```python
from build123d import *

# Parameters (mm, degrees)
BOSS_EXTRUDE1_DEPTH = 20
SKETCH2_R           = 26
CUT_EXTRUDE1_DEPTH  = 5
SKETCH3_R           = 30
CUT_EXTRUDE2_DEPTH  = 11
CUT_EXTRUDE3_DEPTH  = 187.815416923
FILLET1_R           = 6
CHAMFER1_SIZE       = 2
SKETCH6_W           = 10
SKETCH6_H           = 80
CUT_EXTRUDE4_DEPTH  = 5
CHAMFER2_SIZE       = 2
SKETCH7_R           = 10
SKETCH7_R_2         = 20
CUT_EXTRUDE5_DEPTH  = 5
CHAMFER3_SIZE       = 2


with BuildPart() as part:
    # Sketch1 → Boss-Extrude1 (new, symmetric)
    with BuildSketch(Plane.XY):
        with BuildLine():
            Line((-29.941348918, -1.875), (-19.960899278, -161.25))
            ThreePointArc((-19.960899278, -161.25), (0, -180), (19.960899278, -161.25))
            Line((19.960899278, -161.25), (29.941348918, -1.875))
            ThreePointArc((29.941348918, -1.875), (0, 30), (-29.941348918, -1.875))
        make_face()
    extrude(amount=BOSS_EXTRUDE1_DEPTH, both=True)

    # Sketch2 → Cut-Extrude1 (cut)
    with BuildSketch(Plane(origin=(0, 0, -20), x_dir=(-1, 0, 0), z_dir=(0, 0, -1))):
        Circle(SKETCH2_R)
    extrude(amount=-CUT_EXTRUDE1_DEPTH, mode=Mode.SUBTRACT)

    # Sketch3 → Cut-Extrude2 (cut, symmetric)
    with BuildSketch(Plane.XY):
        with Locations((0, -160)):
            Circle(SKETCH3_R)
    extrude(amount=CUT_EXTRUDE2_DEPTH, both=True, mode=Mode.SUBTRACT)

    # Sketch4 → Cut-Extrude3 (cut, through all)
    with BuildSketch(Plane(origin=(0, 0, -20), x_dir=(-1, 0, 0), z_dir=(0, 0, -1))):
        with BuildLine():
            ThreePointArc((-20.17601335, -29.814903745), (0, -36), (20.17601335, -29.814903745))
            Line((20.17601335, -29.814903745), (14.361387571, -122.667031366))
            ThreePointArc((14.361387571, -122.667031366), (0, -120), (-14.361387571, -122.667031366))
            Line((-14.361387571, -122.667031366), (-20.17601335, -29.814903745))
        make_face()
    extrude(amount=-CUT_EXTRUDE3_DEPTH, mode=Mode.SUBTRACT)

    # Fillet1
    fillet1_edges = [part.edges().sort_by_distance(p)[0] for p in [
        (20.17601335, -29.814903745, 0),
        (-20.17601335, -29.814903745, 0),
        (-14.361387571, -122.667031366, 0),
        (14.361387571, -122.667031366, 0),
    ]]
    fillet(fillet1_edges, radius=FILLET1_R)

    # Chamfer1
    chamfer1_edges = [part.edges().sort_by_distance(p)[0] for p in [
        (0, -180, 20),
        (24.951124098, -81.5625, 20),
        (0, 30, 20),
        (24.951124098, -81.5625, -20),
        (0, -120, -20),
        (0, -120, 20),
        (17.178453178, -77.682101085, -20),
        (0, -180, -20),
        (17.178453178, -77.682101085, 20),
        (-17.178453178, -77.682101085, -20),
        (-17.178453178, -77.682101085, 20),
        (-24.951124098, -81.5625, -20),
        (0, -36, -20),
        (0, -36, 20),
        (12.505327982, -119.60645162, -20),
        (12.505327982, -119.60645162, 20),
        (-12.505327982, -119.60645162, -20),
        (-12.505327982, -119.60645162, 20),
        (17.184830058, -34.989739942, -20),
        (0, 30, -20),
        (17.184830058, -34.989739942, 20),
        (-17.184830058, -34.989739942, -20),
        (-17.184830058, -34.989739942, 20),
        (-24.951124098, -81.5625, 20),
    ]]
    chamfer(chamfer1_edges, length=CHAMFER1_SIZE)

    # Sketch6 → Cut-Extrude4 (cut)
    with BuildSketch(Plane(origin=(29.941348918, -1.875, 0), x_dir=(0, 0, -1), z_dir=(0.9980449639169572, -0.06249999999999988, 0))):
        with Locations((0, -60)):
            Rectangle(SKETCH6_W, SKETCH6_H)
    extrude(amount=-CUT_EXTRUDE4_DEPTH, mode=Mode.SUBTRACT)

    # Chamfer2
    chamfer2_edges = [part.edges().sort_by_distance(p)[0] for p in [
        (21.201124098, -61.445197835, 5),
        (23.701124098, -21.523399278, 0),
        (21.201124098, -61.445197835, -5),
        (18.701124098, -101.366996392, 0),
    ]]
    chamfer(chamfer2_edges, length=CHAMFER2_SIZE)

    # Sketch7 → Cut-Extrude5 (cut)
    with BuildSketch(Plane.XY.offset(20)):
        with Locations((0, -160)):
            Circle(SKETCH7_R)
        Circle(SKETCH7_R_2)
    extrude(amount=-CUT_EXTRUDE5_DEPTH, mode=Mode.SUBTRACT)

    # Chamfer3
    chamfer3_edges = [part.edges().sort_by_distance(p)[0] for p in [
        (-10, -160, 15),
        (-10, -160, 20),
        (-20, 0, 15),
        (-20, 0, 20),
    ]]
    chamfer(chamfer3_edges, length=CHAMFER3_SIZE)


solid = part.part
```
The listing builds one solid part. Answer for the finished solid, in the listing's coordinates (mm). A direction names the side the tool comes from. Round coordinates to 2 decimals unless told otherwise and drop trailing zeros. Write each loop counter-clockwise with the first axis right and the second up, starting at its lowest first coordinate (ties: lowest second). Pieces come first, ordered by that corner, then holes. Notation, with made-up numbers: (45, -7.75) -> (64, -7.75) arc R11 ccw to (64, 2.25) -> close; hole circle Ø9 at (-30.75, -37). An arc over 180 degrees is marked (long way). Use CSV: the item, a comma, the result in double quotes. Start each with the question number.
(1) Section A-A on y = -89 is taken. Give the vertices of the cut face in (x, z).
(2) Which of the six approach directions +Z, -Z, +X, -X, +Y, -Y give full straight-line access (tool end or side, diameter ignored) to faces 4 (the face through (18.13, -78.269, 18.986)), 5 (the face through (0, -120, 0)), 6 (the face through (22.15, -62.066, -3.986)), 7 (the face through (20.633, -15.821, -17.535)), 8 (the face through (0, -130, 0))?
(3) Each of these flat-tipped pins is pushed along its axis until it touches: pin 1 (18 mm diameter, centred on x = -4.5, y = -1.5, fed in from +Z); pin 2 (15.5 mm diameter, centred on x = -8, y = -4, fed in from -Z); pin 3 (17.5 mm diameter, centred on x = 3, y = -160, fed in from +Z). Where does it stop, or does it pass through?
(4) Consider L1, parallel to Z at x = -13, y = -168.5; L2, parallel to Y at x = -0.5, z = -13; L3, parallel to Z at x = -18.5, y = -9.5. Determine where each line is inside the solid, lowest interval first. Write a range as from..to.
(5) The mould has two halves that part along X. Classify faces 1 (the face through (12.45, -119.65, 0.25)), 2 (the face through (25, -62, 5)), 3 (the face through (0.65, 28.31, -19.68)): released by +X, released by -X, zero draft, split by the parting line, or undercut.
(6) Section B-B on z = 8 is taken. Give the vertices of the cut face in (x, y) (3 decimals).
A:
1,outline,"(-24.49, -18) -> (-22.48, -20) -> (-18.47, -20) -> (-16.47, -18) -> (-16.47, 18) -> (-18.47, 20) -> (-22.48, 20) -> (-24.49, 18) -> close; (16.47, -18) -> (18.47, -20) -> (22.48, -20) -> (24.49, -18) -> (24.49, -5) -> (21.48, -5) -> (19.48, -3) -> (19.48, 3) -> (21.48, 5) -> (24.49, 5) -> (24.49, 18) -> (22.48, 20) -> (18.47, 20) -> (16.47, 18) -> close"
2,face 4,"+Z"
2,face 5,"+Z, -Z"
2,face 6,"+X"
2,face 7,"-Z"
2,face 8,"-Y"
3,pin 1,"stops at z = 15"
3,pin 2,"stops at z = -15"
3,pin 3,"stops at z = 19.75"
4,L1,"z = -20..-11, 11..20"
4,L2,"y = -179.99..-120, -36..30"
4,L3,"z = -15..18.8"
5,face 1,"undercut"
5,face 2,"zero draft"
5,face 3,"split by the parting line"
6,outline,"(-29.941, -1.875) -> (-21.358, -138.933) arc R30 cw to (21.358, -138.933) -> (29.941, -1.875) arc R30 ccw (long way) to start; hole (-19.53, -40.132) -> (-14.827, -115.232) arc R6 ccw to (-7.686, -120.745) arc R40 cw to (7.686, -120.745) arc R6 ccw to (14.827, -115.232) -> (19.53, -40.132) arc R6 ccw to (11.607, -34.077) arc R36 cw to (-11.607, -34.077) arc R6 ccw to start"
